Autodesk Inventor part; units mm, degrees
ref_plane "YZ Plane" through (0, 0, 0) normal (1, 0, 0) x (0, 1, 0)
ref_plane "XZ Plane" through (0, 0, 0) normal (0, 1, 0) x (-1, 0, 0)
ref_plane "XY Plane" through (0, 0, 0) normal (0, 0, 1) x (1, 0, 0)
sketch "Sketch1" plane through (0, 0, 0) normal (1, 0, 0) x (0, 1, 0)
  circle A0 centre (0, 0) radius 35
  circle A1 centre (0, 0) radius 125
  circle A2 centre (0, 0) radius 10 construction
  line L0 (-8.55, -5.1863) -> (-8.7665, 4.8113)
  line L1 (-8.7665, 4.8113) -> (-0.2165, 9.9977)
  line L2 (-0.2165, 9.9977) -> (8.55, 5.1863)
  line L3 (8.55, 5.1863) -> (8.7665, -4.8113)
  line L4 (8.7665, -4.8113) -> (0.2165, -9.9977)
  line L5 (0.2165, -9.9977) -> (-8.55, -5.1863)
  circle A3 centre (0, 0) radius 15
  circle A4 centre (0, 0) radius 75 construction
  circle A5 centre (75, 0) radius 15
  circle A6 centre (-37.5, 64.9519) radius 15
  circle A7 centre (-37.5, -64.9519) radius 15
  circle A8 centre (0, 0) radius 11
  dimension "d2" = 20
  dimension "d12" = 150
  dimension "d0" = 70
  dimension "d1" = 250
  dimension "d3" = 30
  dimension "d13" = 30
  dimension "d16" = 360
  dimension "d20" = 22
extrude "Extrusion1" add sketch "Sketch1" along normal mid plane 10 contours A0 | A1 | L0 L1 L2 L3 L4 L5 | A3 | A5 | A6 | A7 | A8
extrude "Extrusion2" add sketch "Sketch1" against normal blind 300 contours A0
extrude "Extrusion3" add sketch "Sketch1" along normal blind 15 contours L0 L1 L2 L3 L4 L5
extrude "Extrusion4" add sketch "Sketch1" along normal blind 12 contours A3 | A8
extrude "Extrusion5" cut sketch "Sketch1" along normal through all both and the other way through all contours A5 | A6 | A7
extrude "Extrusion6" add sketch "Sketch1" along normal blind 18 contours L0 L1 L2 L3 L4 L5 | A8
sketch "Sketch2" plane through (-300, 0, 0) normal (-1, 0, 0) x (0, 0, 1)
  circle A0 centre (0, 0) radius 125
  circle A1 centre (0, 75) radius 15
  circle A2 centre (-64.9519, -37.5) radius 15
  circle A3 centre (64.9519, -37.5) radius 15
  circle A4 centre (0, 0) radius 15
  circle A5 centre (0, 0) radius 10
  line L0 (4.8113, -8.7665) -> (-5.1863, -8.55)
  line L1 (-5.1863, -8.55) -> (-9.9977, 0.2165)
  line L2 (-9.9977, 0.2165) -> (-4.8113, 8.7665)
  line L3 (-4.8113, 8.7665) -> (5.1863, 8.55)
  line L4 (5.1863, 8.55) -> (9.9977, -0.2165)
  line L5 (9.9977, -0.2165) -> (4.8113, -8.7665)
extrude "Extrusion7" add sketch "Sketch2" along normal mid plane 10 contours A0
extrude "Extrusion8" add sketch "Sketch2" along normal blind 300 contours A5 L4 | L3 A5 | L4 L5 L0 L1 L2 L3 | A5 L5 | L2 A5 | A5 L0 | L1 A5
extrude "Extrusion10" add sketch "Sketch2" along normal blind 40 contours A4 | A5 L4 | L3 A5 | L4 L5 L0 L1 L2 L3 | A5 L5 | L2 A5 | A5 L0 | L1 A5
properties part number "roller"
The model under review builds one solid part; all positions refer to its coordinate system, in mm. A direction names the side the tool comes from. Round coordinates to 2 decimals unless told otherwise and drop trailing zeros. Loops run counter-clockwise (first coordinate to the right, second up) from the corner with the lowest first, then second, coordinate; pieces in that order, holes last. Notation, with made-up numbers: (11, -22.5) -> (68, -22.5) arc R21 cw to (68, 11.5) -> close; hole circle Ø10 at (72.25, -20). An arc over 180 degrees is marked (long way). Answer as CSV lines item,"result".
1) Add section A-A on y = 75. Write out the cut boundary in (x, z), plus the area to 3 significant figures.
Geometry results:
outline,"(-305, -100) -> (-295, -100) -> (-295, -15) -> (-305, -15) -> close; (-305, 15) -> (-295, 15) -> (-295, 100) -> (-305, 100) -> close; (-5, -100) -> (5, -100) -> (5, -15) -> (-5, -15) -> close; (-5, 15) -> (5, 15) -> (5, 100) -> (-5, 100) -> close"
area,"3,400 mm²"
2) To check wall thickness, follow line 1 along Z through (x, y) = (-88, 0); line 2 along X through (y, z) = (9, -82.5); line 3 along Z through (x, y) = (-297, -37). State the ranges of each line that lie inside material, in increasing order. Write a range as from..to.
Geometry results:
line 1,"z = -35..-15, 15..35"
line 2,"x = -305..-295, -5..5"
line 3,"z = -119.4..-79.94, -49.96..49.96, 79.94..119.4"
3) Tool access review of faces 1 (the face through (-299.93, 89.643, -3.252)), 2 (the face through (-295, -26, 26)), 3 (the face through (14.96, -2.38, 10.74)), 4 (the face through (-322.255, -0.66, -14.985)): name each direction out of +Z, -Z, +X, -X, +Y, -Y from which nothing blocks a thin tool from reaching the whole face with its end or side.
Geometry results:
face 1,"+X, -X"
face 2,"none"
face 3,"+X"
face 4,"-X"
4) For P1, Ø3, axis at x = -93, y = -8.5, coming from the +Z side; P2, Ø5, axis at y = 46.5, z = 59, coming from the +X side, all flat-tipped, find the tip position at first contact; note any pin that passes through.
Geometry results:
P1,"stops at z = 34.29"
P2,"stops at x = 5"
5) Draft analysis for pull direction X (two halves, no side actions). For faces 5 (the face through (18, 0, 0)), 6 (the face through (-5, 0, 0)), 7 (the face through (0.07, -124.88, 5.5)), 8 (the face through (-148, -28, -21)), state which applies: pulls with the +X half, pulls with the -X half, needs draft (parallel to the pull), parting line crosses it, or undercut.
Geometry results:
face 5,"pulls with the +X half"
face 6,"undercut"
face 7,"needs draft"
face 8,"undercut"
6) Add section D-D on y = -85. Write out the cut boundary in (x, z).
Geometry results:
outline,"(-305, -91.65) -> (-295, -91.65) -> (-295, 91.65) -> (-305, 91.65) -> close; (-5, -91.65) -> (5, -91.65) -> (5, 91.65) -> (-5, 91.65) -> close"
7) Add section B-B on z = 0. State how many separate pieces and enclosed holes the cut face has, plus the area to 3 significant figures.
Geometry results:
separate pieces,"3"
enclosed holes,"1"
area,"22,400 mm²"
